Here's how the part is built. I have some questions about the finished solid (model axes, mm). A direction names the side the tool comes from. Round coordinates to 2 decimals unless told otherwise and drop trailing zeros. Write each loop counter-clockwise with the first axis right and the second up, starting at its lowest first coordinate (ties: lowest second). Pieces come first, ordered by that corner, then holes. Notation, with made-up numbers: (58.25, -7.75) -> (68.25, -7.75) arc R24 ccw to (68.25, 27.25) -> close; hole circle Ø5 at (76.5, 58). An arc over 180 degrees is marked (long way). Put each result on its own line as item: value. Start each with the question number.
1) Which directions (+Z, -Z, +X, -X, +Y, -Y) give clear straight access to the entire face, cutting with the end or side of a thin tool? Please do faces 1 (the flat face through (2, -105.74, 5)), 2 (the flat face through (2, 36.26, 5)).
2) We'd pull the mould along X, two halves only. Please class faces 3 (the flat face through (2, -113.74, 5)), 4 (the flat face through (-64.211, -40, 5)), 5 (the flat face through (2, 28.26, 5)), 6 (the flat face through (77.789, -40, 5)): released by +X, released by -X, zero draft, split by the parting line, or undercut.
3) I want a section at B-B, the plane x = 55. List the corners of the cut face in (y, z) for me, then the cut area to 3 significant figures.
4) I want a section at A-A, the plane z = 3.75. List the corners of the cut face in (x, y) for me, then the cut area to 3 significant figures.
5) If I drill on line 1 along X through (y, z) = (-104.5, 9.5); line 2 along Y through (x, z) = (62.5, 8.25), over which ranges is the centre line in solid material (lowest first)? Write a range as [from, to].
6) I want a section at C-C, the plane y = -44.5. List the corners of the cut face in (x, z) for me.
from build123d import *

# Parameters (mm, degrees)
SKETCH1_W           = 150
SKETCH1_H           = 150
BOSS_EXTRUDE1_DEPTH = 10
SKETCH2_W           = 134
SKETCH2_H           = 134
CUT_EXTRUDE1_DEPTH  = 139.158896854
SKETCH3_R           = 1.4
BOSS_EXTRUDE2_DEPTH = 3


with BuildPart() as part:
    # Sketch1 → Boss-Extrude1 (new body)
    with BuildSketch(Plane.XY):
        with Locations((2.789256198, -38.739669421)):
            Rectangle(SKETCH1_W, SKETCH1_H)
    extrude(amount=BOSS_EXTRUDE1_DEPTH)

    # Sketch2 → Cut-Extrude1 (cut, through all)
    with BuildSketch(Plane.XY.offset(10)):
        with Locations((2.789256198, -38.739669421)):
            Rectangle(SKETCH2_W, SKETCH2_H)
    extrude(amount=-CUT_EXTRUDE1_DEPTH, mode=Mode.SUBTRACT)

    # Sketch3 → Boss-Extrude2 (add)
    with BuildSketch(Plane.XY.offset(10)):
        with Locations((73.789256198, -13.739669421)):
            Circle(SKETCH3_R)
        with Locations((27.789256198, -109.739669421)):
            Circle(SKETCH3_R)
        with Locations((-68.210743802, -63.739669421)):
            Circle(SKETCH3_R)
        with Locations((-2.210743802, 32.260330579)):
            Circle(SKETCH3_R)
    extrude(amount=BOSS_EXTRUDE2_DEPTH)


solid = part.part
Findings:
1. face 1: +Z, -Z
1. face 2: +Z, -Z, +X, -X, +Y
2. face 3: zero draft
2. face 4: undercut
2. face 5: undercut
2. face 6: released by +X
3. outline: (-113.74, 0) -> (-105.74, 0) -> (-105.74, 10) -> (-113.74, 10) -> close; (28.26, 0) -> (36.26, 0) -> (36.26, 10) -> (28.26, 10) -> close
3. area: 160 mm2
4. outline: (-72.21, -113.74) -> (77.79, -113.74) -> (77.79, 36.26) -> (-72.21, 36.26) -> close; hole (-64.21, -105.74) -> (69.79, -105.74) -> (69.79, 28.26) -> (-64.21, 28.26) -> close
4. area: 4,540 mm2
5. line 1: x = [-72.21, -64.21], [69.79, 77.79]
5. line 2: y = [-113.74, -105.74], [28.26, 36.26]
6. outline: (-72.21, 0) -> (-64.21, 0) -> (-64.21, 10) -> (-72.21, 10) -> close; (69.79, 0) -> (77.79, 0) -> (77.79, 10) -> (69.79, 10) -> close
